Can you work these out from the drawing? Everything is in mm from the part's minimum corner. Coordinates: 2 decimals unless noted, no trailing zeros. Loops run counter-clockwise (first coordinate to the right, second up) from the corner with the lowest first, then second, coordinate; pieces in that order, holes last.
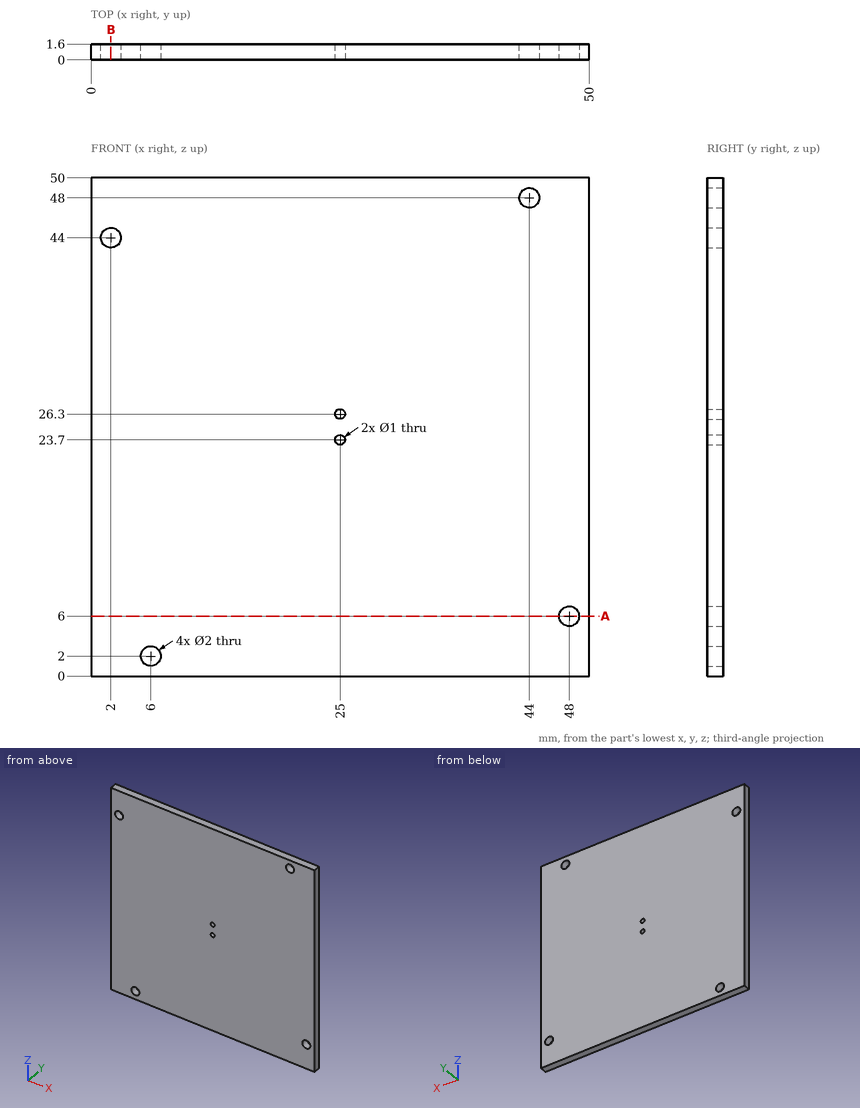
Item 1: Suppose I cut it at B-B, the plane x = 2. Please give me the cut outline in (y, z).
Results are:
outline: (0, 0) - (1.6, 0) - (1.6, 43) - (0, 43) - close; (0, 45) - (1.6, 45) - (1.6, 50) - (0, 50) - close
Item 2: I'm going to push a flat-ended pin straight in: P1, Ø1.6, axis at x = 48, z = 6, coming from the +Y side. Where does the tip first touch, or does it pass through?
Results are:
P1: passes through
Item 3: I need wall thicknesses on line 1 along Z through (x, y) = (25, 1.2); line 2 along Z through (x, y) = (6, 0.9); line 3 along X through (y, z) = (0.4, 48). Which ranges of each line are inside material? Lowest first, please.
Results are:
line 1: z = 0 to 23.2, 24.2 to 25.8, 26.8 to 50
line 2: z = 0 to 1, 3 to 50
line 3: x = 0 to 43, 45 to 50
Item 4: Suppose I cut it at A-A, the plane z = 6. Please give me the cut outline in (x, y).
Results are:
outline: (0, 0) - (47, 0) - (47, 1.6) - (0, 1.6) - close; (49, 0) - (50, 0) - (50, 1.6) - (49, 1.6) - close
